Check sheet for the modelled part. Datum: model origin and axes. Units: mm. A direction names the side the tool comes from. Round coordinates to 2 decimals unless told otherwise and drop trailing zeros. Order: outer loops, then holes, each group sorted by start corner. A loop starts at its lowest first (then second) coordinate and runs counter-clockwise, first axis right, second up.
Q1. Depth check by flat-ended pin: P1, Ø3, axis at x = 8.5, y = 17, coming from the -Z side; P2, Ø2.5, axis at x = 1.5, z = -2, coming from the +Y side; P3, Ø6.5, axis at x = -59.5, z = -41.5, coming from the +Y side. Enter the tip coordinate at first touch or a pass-through.
Q2. Cross-section at C-C on z = 53.5. Record the cut outline in (x, y).
Q3. Scan lines: probe 1 along X at (y, z) = (47.25, -43); probe 2 along X at (y, z) = (29.5, -46.5); probe 3 along X at (y, z) = (47, 24). Record each from-to range of solid material in increasing order.
Q4. Cross-section at D-D on z = 11. Record the cut outline in (x, y), then the cut area to 3 significant figures.
Q5. Cross-section at B-B on x = -32. Record the cut outline in (y, z), then the cut area to 3 significant figures.
Q6. Cross-section at A-A on z = -27.5. Record the cut outline in (x, y), then the cut area to 3 significant figures.
Q7. Mould release check, pull along Z, two halves, no side actions. Record for faces 4 (the flat face through (-1, 4, 6)), 5 (the flat face through (-1, 0, -8)), 6 (the flat face through (55, 48, -43)), 7 (the flat face through (-45, 27, -76.5)): +Z half, -Z half, draft (parallel to the pull), parting line (faces both ways), or undercut.
Q8. Set-up check for faces 1 (the flat face through (65, 29, -1)), 2 (the flat face through (-67, 27, -9.817)), 3 (the flat face through (3, 23.5, -2)): record each of +Z, -Z, +X, -X, +Y, -Y from which the full face is reachable in a straight line by a thin tool's end or side.
from build123d import *

# Parameters (mm, degrees)
BOSS_EXTRUDE1_DEPTH = 4
BOSS_EXTRUDE2_START = 4
BOSS_EXTRUDE2_DEPTH = 50
SKETCH3_R           = 7.5
SKETCH3_R_2         = 1.5
BOSS_EXTRUDE3_DEPTH = 19.5
SKETCH4_W           = 13
SKETCH4_H           = 7
BOSS_EXTRUDE4_DEPTH = 17.81
SKETCH5_W           = 13
SKETCH5_H           = 7
BOSS_EXTRUDE5_DEPTH = 10
CUT_EXTRUDE1_REACH  = 117.087
SKETCH6_R           = 1.5
CUT_EXTRUDE2_REACH  = 149.777
SKETCH7_W           = 32
SKETCH7_H           = 28
CUT_EXTRUDE3_REACH  = 165.476
SKETCH8_W           = 33
SKETCH8_H           = 8
SKETCH8_W_2         = 28.7
SKETCH8_H_2         = 5


with BuildPart() as part:
    # Sketch1 → Boss-Extrude1 (new body)
    with BuildSketch(Plane(origin=(0, 0, 0), x_dir=(1, 0, 0), z_dir=(0, 1, 0))):
        Polygon((-69, -61.5), (69, -61.5), (69, 61.5), (-21, 61.5), (-21, 76.5), (-69, 76.5), (-69, 61.5), align=None)
    extrude(amount=BOSS_EXTRUDE1_DEPTH)

    # Sketch1<5> → Boss-Extrude2 (add)
    with BuildSketch(Plane(origin=(0, 0, 0), x_dir=(1, 0, 0), z_dir=(0, 1, 0)).offset(BOSS_EXTRUDE2_START)):
        Polygon((-69, 61.5), (-69, -61.5), (69, -61.5), (69, 61.5), (-21, 61.5), (-21, 76.5), (-69, 76.5), align=None)
        Polygon((-65, -57.5), (-65, 57.5), (-65, 72.5), (-24.92925867, 72.5), (-24.92925867, 57.5), (65, 57.5), (65, -57.5), align=None, mode=Mode.SUBTRACT)
    extrude(amount=BOSS_EXTRUDE2_DEPTH)

    # Sketch3 → Boss-Extrude3 (add)
    # profile 1 of 2: a face of its own
    with BuildSketch(Plane(origin=(0, 4, 0), x_dir=(1, 0, 0), z_dir=(0, 1, 0))):
        with Locations(Location((-46.862948708, 2.10374449, 0), (0, 0, 270))):
            Circle(SKETCH3_R)
        with Locations(Location((-46.862948708, 2.10374449, 0), (0, 0, 270))):
            Circle(SKETCH3_R_2, mode=Mode.SUBTRACT)
    # profile 2 of 2: a face of its own
    with BuildSketch(Plane(origin=(0, 4, 0), x_dir=(1, 0, 0), z_dir=(0, 1, 0))):
        with Locations(Location((1.137051292, 2.10374449, 0), (0, 0, 270))):
            Circle(SKETCH3_R)
        with Locations(Location((1.137051292, 2.10374449, 0), (0, 0, 270))):
            Circle(SKETCH3_R_2, mode=Mode.SUBTRACT)
    extrude(amount=BOSS_EXTRUDE3_DEPTH)

    # Sketch4 → Boss-Extrude4 (add)
    with BuildSketch(Plane(origin=(-65, 0, 0), x_dir=(0, 0, -1), z_dir=(1, 0, 0))):
        with Locations((-24.47, 47.8)):
            Rectangle(SKETCH4_W, SKETCH4_H)
        with Locations((43, 47.8)):
            Rectangle(SKETCH4_W, SKETCH4_H)
    extrude(amount=BOSS_EXTRUDE4_DEPTH)

    # Sketch5 → Boss-Extrude5 (add)
    with BuildSketch(Plane.ZY.offset(-65)):
        with Locations((24.47, 47.8)):
            Rectangle(SKETCH5_W, SKETCH5_H)
        with Locations((-43, 47.8)):
            Rectangle(SKETCH5_W, SKETCH5_H)
    extrude(amount=BOSS_EXTRUDE5_DEPTH)

    # Sketch6 → Cut-Extrude1 (cut, up to next)
    with BuildSketch(Plane(origin=(0, 51.3, 0), x_dir=(1, 0, 0), z_dir=(0, 1, 0)), mode=Mode.PRIVATE) as cut_extrude1_sk1:
        with Locations(Location((-53.69, 43, 0), (0, 0, 270))):
            Circle(SKETCH6_R)
    cut_extrude1_tool1 = extrude(cut_extrude1_sk1.sketch, amount=-CUT_EXTRUDE1_REACH, mode=Mode.PRIVATE) & part.part
    # Sketch6 → Cut-Extrude1 (cut, up to next)
    with BuildSketch(Plane(origin=(0, 51.3, 0), x_dir=(1, 0, 0), z_dir=(0, 1, 0)), mode=Mode.PRIVATE) as cut_extrude1_sk2:
        with Locations(Location((-53.69, -24.47, 0), (0, 0, 270))):
            Circle(SKETCH6_R)
    cut_extrude1_tool2 = extrude(cut_extrude1_sk2.sketch, amount=-CUT_EXTRUDE1_REACH, mode=Mode.PRIVATE) & part.part
    # Sketch6 → Cut-Extrude1 (cut, up to next)
    with BuildSketch(Plane(origin=(0, 51.3, 0), x_dir=(1, 0, 0), z_dir=(0, 1, 0)), mode=Mode.PRIVATE) as cut_extrude1_sk3:
        with Locations(Location((60, -24.47, 0), (0, 0, 270))):
            Circle(SKETCH6_R)
    cut_extrude1_tool3 = extrude(cut_extrude1_sk3.sketch, amount=-CUT_EXTRUDE1_REACH, mode=Mode.PRIVATE) & part.part
    # Sketch6 → Cut-Extrude1 (cut, up to next)
    with BuildSketch(Plane(origin=(0, 51.3, 0), x_dir=(1, 0, 0), z_dir=(0, 1, 0)), mode=Mode.PRIVATE) as cut_extrude1_sk4:
        with Locations(Location((60, 43, 0), (0, 0, 270))):
            Circle(SKETCH6_R)
    cut_extrude1_tool4 = extrude(cut_extrude1_sk4.sketch, amount=-CUT_EXTRUDE1_REACH, mode=Mode.PRIVATE) & part.part
    add(cut_extrude1_tool1.solids().sort_by_distance((-53.69, 51.3, -43))[0], mode=Mode.SUBTRACT)
    add(cut_extrude1_tool2.solids().sort_by_distance((-53.69, 51.3, 24.47))[0], mode=Mode.SUBTRACT)
    add(cut_extrude1_tool3.solids().sort_by_distance((60, 51.3, 24.47))[0], mode=Mode.SUBTRACT)
    add(cut_extrude1_tool4.solids().sort_by_distance((60, 51.3, -43))[0], mode=Mode.SUBTRACT)

    # Sketch7 → Cut-Extrude2 (cut, up to next)
    with BuildSketch(Plane.XY.offset(-57.5), mode=Mode.PRIVATE) as cut_extrude2_sk1:
        with Locations((12.5, 40)):
            Rectangle(SKETCH7_W, SKETCH7_H)
    cut_extrude2_tool1 = extrude(cut_extrude2_sk1.sketch, amount=-CUT_EXTRUDE2_REACH, mode=Mode.PRIVATE) & part.part
    add(cut_extrude2_tool1.solids().sort_by_distance((12.5, 40, -57.5))[0], mode=Mode.SUBTRACT)

    # Sketch8 → Cut-Extrude3 (cut, up to next)
    with BuildSketch(Plane(origin=(-65, 0, 0), x_dir=(0, 0, -1), z_dir=(1, 0, 0)), mode=Mode.PRIVATE) as cut_extrude3_sk1:
        with Locations((-22, 38)):
            Rectangle(SKETCH8_W, SKETCH8_H)
    cut_extrude3_tool1 = extrude(cut_extrude3_sk1.sketch, amount=-CUT_EXTRUDE3_REACH, mode=Mode.PRIVATE) & part.part
    # Sketch8 → Cut-Extrude3 (cut, up to next)
    with BuildSketch(Plane(origin=(-65, 0, 0), x_dir=(0, 0, -1), z_dir=(1, 0, 0)), mode=Mode.PRIVATE) as cut_extrude3_sk2:
        with Locations((24.167352626, 27.5)):
            Rectangle(SKETCH8_W_2, SKETCH8_H_2)
    cut_extrude3_tool2 = extrude(cut_extrude3_sk2.sketch, amount=-CUT_EXTRUDE3_REACH, mode=Mode.PRIVATE) & part.part
    add(cut_extrude3_tool1.solids().sort_by_distance((-65, 38, 22))[0], mode=Mode.SUBTRACT)
    add(cut_extrude3_tool2.solids().sort_by_distance((-65, 27.5, -24.167353))[0], mode=Mode.SUBTRACT)


solid = part.part
Results found:
1. P1: stops at z = -61.5
1. P2: stops at y = 23.5
1. P3: stops at y = 51.3
2. outline: (-69, 0) - (69, 0) - (69, 54) - (65, 54) - (65, 4) - (-65, 4) - (-65, 54) - (-69, 54) - close
3. probe 1: x = -69 to -55.19, -52.19 to -47.19, 55 to 58.5, 61.5 to 69
3. probe 2: x = -69 to -65, 65 to 69
3. probe 3: x = -69 to -55.11, -52.27 to -47.19, 55 to 58.58, 61.42 to 69
4. outline: (-69, 0) - (69, 0) - (69, 54) - (65, 54) - (65, 4) - (-65, 4) - (-65, 34) - (-69, 34) - close; (-69, 42) - (-65, 42) - (-65, 54) - (-69, 54) - close
4. area: 920 mm2
5. outline: (0, -76.5) - (54, -76.5) - (54, -72.5) - (4, -72.5) - (4, 57.5) - (54, 57.5) - (54, 61.5) - (0, 61.5) - close
5. area: 952 mm2
6. outline: (-69, 0) - (69, 0) - (69, 54) - (65, 54) - (65, 4) - (-65, 4) - (-65, 25) - (-69, 25) - close; (-69, 30) - (-65, 30) - (-65, 54) - (-69, 54) - close
6. area: 932 mm2
7. face 4: undercut
7. face 5: draft
7. face 6: undercut
7. face 7: -Z half
8. face 1: none
8. face 2: -X
8. face 3: +Y
